For this review, use the dimensioned drawing (mm, ordinates from the lowest corner) and the shaded views. Give positions to 0.01 mm unless a question says otherwise; leave off trailing zeros. Write each loop counter-clockwise with the first axis right and the second up, starting at its lowest first coordinate (ties: lowest second). Pieces come first, ordered by that corner, then holes. Notation, with made-up numbers: (47, 2) -> (59, 2) arc R12 cw to (59, 16) -> close; hole circle Ø4 at (60, 19). An arc over 180 degrees is marked (long way). Write each question's results on one line, items separated by ' | '. Start each with the question number.
(1) Take a section at A-A (y = 12.5). State the section outline as (x, z) points.
(2) Take a section at B-B (x = 15). State the section outline as (y, z) points.
(3) Clearance check with a flat-ended pin moving along its axis: pin 1 (2.5 mm diameter, centred on y = 16.5, z = 12, fed in from +X). State where the tip first meets the part, or that it passes through.
(4) To check wall thickness, follow probe 1 along X at (y, z) = (13, 22.25) (1 decimal); probe 2 along Y at (x, z) = (15, 18.5); probe 3 along X at (y, z) = (10.75, 17). State the ranges of each line that lie inside material, in increasing order.
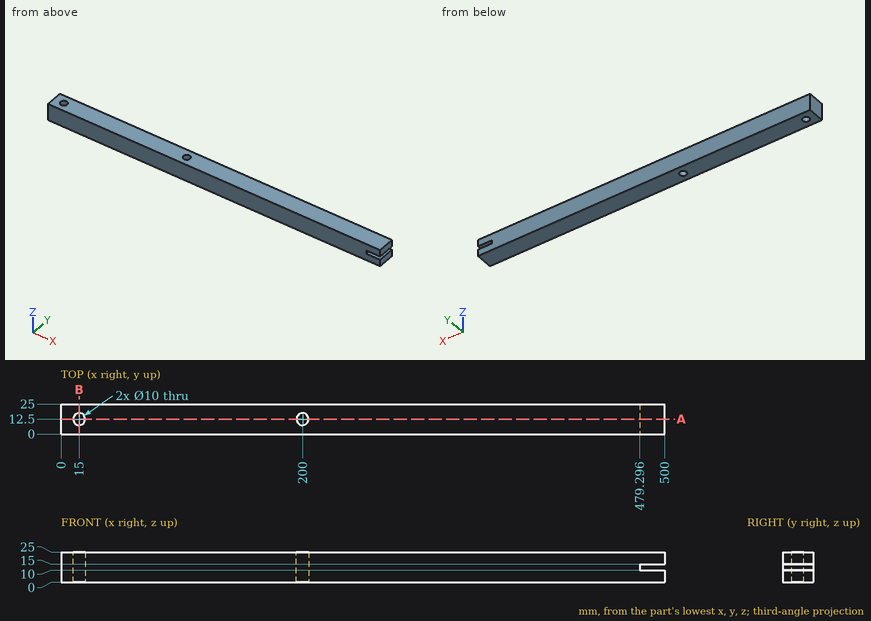
Report:
1) outline: (0, 0) -> (10, 0) -> (10, 25) -> (0, 25) -> close; (20, 0) -> (195, 0) -> (195, 25) -> (20, 25) -> close; (205, 0) -> (500, 0) -> (500, 10) -> (479.3, 10) -> (479.3, 15) -> (500, 15) -> (500, 25) -> (205, 25) -> close
2) outline: (0, 0) -> (7.5, 0) -> (7.5, 25) -> (0, 25) -> close; (17.5, 0) -> (25, 0) -> (25, 25) -> (17.5, 25) -> close
3) pin 1: x = 479.3
4) probe 1: 0 to 10, 20 to 195, 205 to 500 | probe 2: 0 to 7.5, 17.5 to 25 | probe 3: 0 to 10.32, 19.68 to 195.32, 204.68 to 500
